```python
from build123d import *

# Parameters (mm, degrees)
SKETCH2_R                 = 25
SKETCH2_R_2               = 19
BOSS_EXTRUDE1_DEPTH       = 70
BOSS_EXTRUDE2_START       = 10
SKETCH3_R                 = 38.05
SKETCH3_R_2               = 32.6
BOSS_EXTRUDE2_DEPTH       = 50
BOSS_EXTRUDE3_START       = -50
BOSS_EXTRUDE3_OUTLINE_R   = 39.3
BOSS_EXTRUDE3_OUTLINE_R_2 = 38.05
BOSS_EXTRUDE3_DEPTH       = 10
CUT_EXTRUDE1_REACH        = 162.207
CUT_EXTRUDE1_END_RADIUS   = 32.6
SKETCH7_R                 = 3
CIRPATTERN1_COUNT         = 4


with BuildPart() as part:
    # Sketch2 → Boss-Extrude1 (new body)
    with BuildSketch(Plane(origin=(0, 0, 0), x_dir=(1, 0, 0), z_dir=(0, 1, 0))):
        with Locations(Location((0, 0, 0), (0, 0, 270))):
            Circle(SKETCH2_R)
        with Locations(Location((0, 0, 0), (0, 0, 270))):
            Circle(SKETCH2_R_2, mode=Mode.SUBTRACT)
    extrude(amount=BOSS_EXTRUDE1_DEPTH)



with BuildPart() as body_2:
    # Sketch3 → Boss-Extrude2 (new body)
    with BuildSketch(Plane(origin=(0, 70, 0), x_dir=(1, 0, 0), z_dir=(0, 1, 0)).offset(BOSS_EXTRUDE2_START)):
        with Locations(Location((0, 0, 0), (0, 0, 270))):
            Circle(SKETCH3_R)
        with Locations(Location((0, 0, 0), (0, 0, 270))):
            Circle(SKETCH3_R_2, mode=Mode.SUBTRACT)
    extrude(amount=BOSS_EXTRUDE2_DEPTH)


with BuildPart() as part_1:
    add(part.part)

    add(body_2.part)  # loft3 joins it to this body
    # loft up to a face of the part (loft3)
    loft([Face(Wire([part_1.edges().sort_by_distance((18.224215686, 70, -17.113677648))[0]])), Face(Wire([part_1.edges().sort_by_distance((-27.737256273, 80, -26.047017381))[0]]))])

    # Cut-Loft1: read off the stored shape, not the designer's step
    # Cut-Loft1: loft between two sections, ruled curve by curve
    cut_loft1_from = [
        Edge.make_bspline([(-18.095722376, 70, 5.791790025), (-6.512142325, 70, 41.983234777), (29.679302426, 70, 30.399654727), (18.095722376, 70, -5.791790025), (6.512142325, 70, -41.983234777), (-29.679302426, 70, -30.399654727), (-18.095722376, 70, 5.791790025)], [0, 0, 0, 0, 0.5, 0.5, 0.5, 1, 1, 1, 1], 3, [1, 0.333333333, 0.333333333, 1, 0.333333333, 0.333333333, 1]),
    ]
    cut_loft1_to = [
        Edge.make_bspline([(-21.296342667, 80, 24.682499651), (28.068656636, 80, 67.275184984), (70.661341969, 80, 17.910185682), (21.296342667, 80, -24.682499651), (-28.068656636, 80, -67.275184984), (-70.661341969, 80, -17.910185682), (-21.296342667, 80, 24.682499651)], [0, 0, 0, 0, 0.5, 0.5, 0.5, 1, 1, 1, 1], 3, [1, 0.333333333, 0.333333333, 1, 0.333333333, 0.333333333, 1]),
    ]
    cut_loft1 = Solid(Shell([*[Face.make_surface_from_curves(cut_loft1_from[k], cut_loft1_to[k]) for k in range(1)], Face(Wire(cut_loft1_from)), Face(Wire(cut_loft1_to))]))
    add(cut_loft1, mode=Mode.SUBTRACT)

    # Boss-Extrude3: read off the stored shape, not the designer's step
    # Boss-Extrude3 outline → Boss-Extrude3 (add)
    with BuildSketch(Plane(origin=(0, 130, 0), x_dir=(1, 0, 0), z_dir=(0, 1, 0)).offset(BOSS_EXTRUDE3_START)):
        Circle(BOSS_EXTRUDE3_OUTLINE_R)
        Circle(BOSS_EXTRUDE3_OUTLINE_R_2, mode=Mode.SUBTRACT)
    extrude(amount=BOSS_EXTRUDE3_DEPTH)

    # Cut-Extrude1: up to this cylinder (the profile starts outside it)
    cut_extrude1_end = Plane(origin=(0, 110, 0), z_dir=(0, -1, 0)) * Cylinder(CUT_EXTRUDE1_END_RADIUS, 390.614, mode=Mode.PRIVATE)
    # Sketch7 → Cut-Extrude1 (cut, up to the surface)
    with BuildSketch(Plane(origin=(-26.905413024, 0, 26.905413024), x_dir=(0, -1, 0), z_dir=(-0.7071067811865488, 0, 0.7071067811865464)), mode=Mode.PRIVATE) as cut_extrude1_sk1:
        with Locations(Location((-110, 0, 0), (0, 0, 90))):
            Circle(SKETCH7_R)
    cut_extrude1_tool1 = extrude(cut_extrude1_sk1.sketch, amount=-CUT_EXTRUDE1_REACH, mode=Mode.PRIVATE) - cut_extrude1_end
    cut_extrude1 = cut_extrude1_tool1.solids().sort_by_distance((-26.905413, 110, 26.905413))[0]
    add(cut_extrude1, mode=Mode.SUBTRACT)

    # CirPattern1: Cut-Extrude1 ×4 about axis
    cirpattern1_axis = Axis((0, 130, 0), (0, -1, 0))
    for i in range(1, CIRPATTERN1_COUNT):
        add(cut_extrude1.rotate(cirpattern1_axis, i * 360 / CIRPATTERN1_COUNT), mode=Mode.SUBTRACT)


solid = part_1.part
```
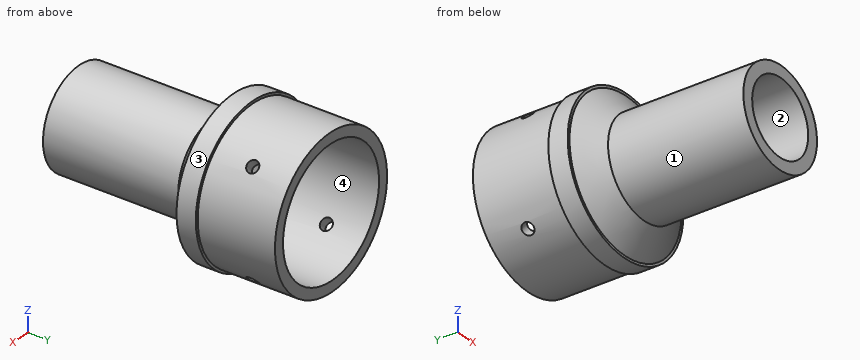
Model file for the job. Use its own axes, mm. Face numbers are marked on the shaded views. A direction names the side the tool comes from. Coordinates: 2 decimals unless noted, no trailing zeros. Order: outer loops, then holes, each group sorted by start corner. A loop starts at its lowest first (then second) coordinate and runs counter-clockwise, first axis right, second up. Notation, with made-up numbers: (11.5, 28.5) -> (39.5, 28.5) arc R26 ccw to (39.5, 61.5) -> close; hole circle Ø4 at (78.25, 69.5). An arc over 180 degrees is marked (long way). Return JSON: item names as keys, results as strings.
Item 1: 3-axis set-ups, long thin cutter, end or side, ignore diameter. For the marked faces 3 and 4: which of +Z, -Z, +X, -X, +Y, -Y reach the whole face in a straight line?
Model answer:
{"face 3": "+Y, -Y", "face 4": "+Y"}
Item 2: Pin check, flat tips, straight feed: P1, Ø10, axis at y = 115, z = -6, coming from the -X side; P2, Ø10, axis at y = 32.5, z = 6.5, coming from the -X side; P3, Ø1, axis at y = 59.5, z = -21.5, coming from the +X side. Stop position of each tip, or through.
Model answer:
{"P1": "stops at x = -38.04", "P2": "stops at x = -24.95", "P3": "stops at x = 13.56"}
Item 3: Slice it at A-A (y = 18). Write the cut outline in (x, z).
Model answer:
{"outline": "circle Ø50 at (0, 0); hole circle Ø38 at (0, 0)"}
Item 4: Wall check: line 1 along Z through (x, y) = (0, 117.5); line 2 along X through (y, z) = (47, 0); line 3 along Z through (x, y) = (1, 56.5). Give the ranges that are in metal, low to high. Write a range as from..to.
Model answer:
{"line 1": "z = -38.05..-32.6, 32.6..38.05", "line 2": "x = -25..-19, 19..25", "line 3": "z = -24.98..-18.97, 18.97..24.98"}
Item 5: Slice it at B-B (y = 118). Write the cut outline in (x, z).
Model answer:
{"outline": "circle Ø76.1 at (0, 0); hole circle Ø65.2 at (0, 0)"}
Item 6: Mould opens along X. For the marked faces 1 and 2 say: pulls with the +X half, pulls with the -X half, needs draft (parallel to the pull), parting line crosses it, or undercut.
Model answer:
{"face 1": "parting line crosses it", "face 2": "undercut"}
